Geometry: final body of the model. Coordinates: model frame, mm. A direction names the side the tool comes from. Round coordinates to 2 decimals unless told otherwise and drop trailing zeros. Loops run counter-clockwise (first coordinate to the right, second up) from the corner with the lowest first, then second, coordinate; pieces in that order, holes last. Notation, with made-up numbers: M 62.25,-9 L 120.25,-9 A19 cw 120.25,-3 Z; hole C 88.25,-6 d10. An arc over 180 degrees is marked long. Write each question's results on one line, items separated by ' | '.
```python
from build123d import *

# Parameters (mm, degrees)
SKETCH1_R           = 13
SKETCH1_R_2         = 9.5
SKETCH1_R_3         = 0.4
BOSS_EXTRUDE1_DEPTH = 1.5
BOSS_EXTRUDE2_DEPTH = 2


with BuildPart() as part:
    # Sketch1 → Boss-Extrude1 (new body)
    with BuildSketch(Plane(origin=(0, 0, 0), x_dir=(1, 0, 0), z_dir=(0, 1, 0))):
        with Locations(Location((0, 0, 0), (0, 0, 270))):
            Circle(SKETCH1_R)
        with Locations(Location((0, 0, 0), (0, 0, 270))):
            Circle(SKETCH1_R_2, mode=Mode.SUBTRACT)
        with Locations(Location((10.5, 0, 0), (0, 0, 270))):
            Circle(SKETCH1_R_3, mode=Mode.SUBTRACT)
        with Locations(Location((9.986093421, -3.244678441, 0), (0, 0, 270))):
            Circle(SKETCH1_R_3, mode=Mode.SUBTRACT)
        with Locations(Location((8.494678441, -6.171745149, 0), (0, 0, 270))):
            Circle(SKETCH1_R_3, mode=Mode.SUBTRACT)
        with Locations(Location((6.171745149, -8.494678441, 0), (0, 0, 270))):
            Circle(SKETCH1_R_3, mode=Mode.SUBTRACT)
        with Locations(Location((3.244678441, -9.986093421, 0), (0, 0, 270))):
            Circle(SKETCH1_R_3, mode=Mode.SUBTRACT)
        with Locations(Location((0, -10.5, 0), (0, 0, 270))):
            Circle(SKETCH1_R_3, mode=Mode.SUBTRACT)
        with Locations(Location((-3.244678441, -9.986093421, 0), (0, 0, 270))):
            Circle(SKETCH1_R_3, mode=Mode.SUBTRACT)
        with Locations(Location((-6.171745149, -8.494678441, 0), (0, 0, 270))):
            Circle(SKETCH1_R_3, mode=Mode.SUBTRACT)
        with Locations(Location((-8.494678441, -6.171745149, 0), (0, 0, 270))):
            Circle(SKETCH1_R_3, mode=Mode.SUBTRACT)
        with Locations(Location((-9.986093421, -3.244678441, 0), (0, 0, 270))):
            Circle(SKETCH1_R_3, mode=Mode.SUBTRACT)
        with Locations(Location((-10.5, 0, 0), (0, 0, 270))):
            Circle(SKETCH1_R_3, mode=Mode.SUBTRACT)
        with Locations(Location((-9.986093421, 3.244678441, 0), (0, 0, 270))):
            Circle(SKETCH1_R_3, mode=Mode.SUBTRACT)
        with Locations(Location((-8.494678441, 6.171745149, 0), (0, 0, 270))):
            Circle(SKETCH1_R_3, mode=Mode.SUBTRACT)
        with Locations(Location((-6.171745149, 8.494678441, 0), (0, 0, 270))):
            Circle(SKETCH1_R_3, mode=Mode.SUBTRACT)
        with Locations(Location((-3.244678441, 9.986093421, 0), (0, 0, 270))):
            Circle(SKETCH1_R_3, mode=Mode.SUBTRACT)
        with Locations(Location((0, 10.5, 0), (0, 0, 270))):
            Circle(SKETCH1_R_3, mode=Mode.SUBTRACT)
        with Locations(Location((3.244678441, 9.986093421, 0), (0, 0, 270))):
            Circle(SKETCH1_R_3, mode=Mode.SUBTRACT)
        with Locations(Location((6.171745149, 8.494678441, 0), (0, 0, 270))):
            Circle(SKETCH1_R_3, mode=Mode.SUBTRACT)
        with Locations(Location((8.494678441, 6.171745149, 0), (0, 0, 270))):
            Circle(SKETCH1_R_3, mode=Mode.SUBTRACT)
        with Locations(Location((9.986093421, 3.244678441, 0), (0, 0, 270))):
            Circle(SKETCH1_R_3, mode=Mode.SUBTRACT)
    extrude(amount=BOSS_EXTRUDE1_DEPTH)

    # Sketch2 → Boss-Extrude2 (add)
    with BuildSketch(Plane(origin=(0, 0, 0), x_dir=(1, 0, 0), z_dir=(0, 1, 0))):
        with BuildLine():
            Line((11.989578808, 0.5), (10.988630488, 0.5))
            ThreePointArc((10.988630488, 0.5), (7.778174593, 7.778174593), (0.5, 10.988630488))
            Line((0.5, 10.988630488), (0.5, 11.989578808))
            ThreePointArc((0.5, 11.989578808), (8.485281374, 8.485281374), (11.989578808, 0.5))
        make_face()
        with BuildLine():
            Line((11.989578808, -0.5), (10.988630488, -0.5))
            ThreePointArc((10.988630488, -0.5), (7.778174593, -7.778174593), (0.5, -10.988630488))
            Line((0.5, -10.988630488), (0.5, -11.989578808))
            ThreePointArc((0.5, -11.989578808), (8.485281374, -8.485281374), (11.989578808, -0.5))
        make_face()
        with BuildLine():
            Line((-0.5, -11.989578808), (-0.5, -10.988630488))
            ThreePointArc((-0.5, -10.988630488), (-7.778174593, -7.778174593), (-10.988630488, -0.5))
            Line((-10.988630488, -0.5), (-11.989578808, -0.5))
            ThreePointArc((-11.989578808, -0.5), (-8.485281374, -8.485281374), (-0.5, -11.989578808))
        make_face()
        with BuildLine():
            Line((-0.5, 10.988630488), (-0.5, 11.989578808))
            ThreePointArc((-0.5, 11.989578808), (-8.485281374, 8.485281374), (-11.989578808, 0.5))
            Line((-11.989578808, 0.5), (-10.988630488, 0.5))
            ThreePointArc((-10.988630488, 0.5), (-7.778174593, 7.778174593), (-0.5, 10.988630488))
        make_face()
    extrude(amount=-BOSS_EXTRUDE2_DEPTH)


solid = part.part
```
1. Section A-A (y = -1.2). Output: boundary loops of the cut face in (x, z), then the cut area to 3 significant figures.
Answer key:
outline: M -11.99,-0.5 A12 ccw -0.5,-11.99 L -0.5,-10.99 A11 cw -10.99,-0.5 Z; M -11.99,0.5 L -10.99,0.5 A11 cw -0.5,10.99 L -0.5,11.99 A12 ccw Z; M 0.5,-11.99 A12 ccw 11.99,-0.5 L 10.99,-0.5 A11 cw 0.5,-10.99 Z; M 0.5,10.99 A11 cw 10.99,0.5 L 11.99,0.5 A12 ccw 0.5,11.99 Z | area: 68.3 mm²
2. Section C-C (z = -7.25). Output: boundary loops of the cut face in (x, y), then the cut area to 3 significant figures.
Answer key:
outline: M -10.79,0 L -9.56,0 L -9.56,-2 L -8.27,-2 L -8.27,0 L -6.14,0 L -6.14,1.5 L -10.79,1.5 Z; M 6.14,0 L 8.27,0 L 8.27,-2 L 9.56,-2 L 9.56,0 L 10.79,0 L 10.79,1.5 L 6.14,1.5 Z | area: 19.1 mm²
3. Access query for faces 4 (the face through (-11.5, -1, 0.5)), 5 (the face through (7.858, -0.986, 7.697)), 6 (the face through (-0.5, -1, -11.5)), 7 (the face through (-7.91, 0.74, -10.316)). Directions: +Z, -Z, +X, -X, +Y, -Y. A direction counts if a zero-diameter tool reaches every point of the face in a straight line with its end or side. Return the directions, or none.
Answer key:
face 4: +X, -X, -Y | face 5: -Y | face 6: +Z, -Z, -Y | face 7: +Y, -Y
4. Section D-D (x = 7). Output: boundary loops of the cut face in (y, z), then the cut area to 3 significant figures.
Answer key:
outline: M -2,-9.75 L 0,-9.75 L 0,-10.95 L 1.5,-10.95 L 1.5,-6.42 L 0,-6.42 L 0,-8.49 L -2,-8.49 Z; M -2,8.49 L 0,8.49 L 0,6.42 L 1.5,6.42 L 1.5,10.95 L 0,10.95 L 0,9.75 L -2,9.75 Z | area: 18.6 mm²
5. Pin query (flat end, axial travel): P1, Ø0.8, axis at y = -1.5, z = -11.5, coming from the +X side; P2, Ø2, axis at y = 1, z = 3, coming from the +X side; P3, Ø1.5, axis at x = 1.5, z = 7.5, coming from the +Y side; P4, Ø0.8, axis at y = -1.5, z = 11.5, coming from the -X side. Return the tip coordinate at first contact, or that it passes through.
Answer key:
P1: stops at x = 4.56 | P2: stops at x = 12.85 | P3: passes through | P4: stops at x = -4.56
6. Draft query along Z for faces 1 (the face through (-8.57, -0.99, 8.4)), 2 (the face through (-6.052, 0.74, 8.876)), 3 (the face through (-8, -2, -8)). Return one class per face: pulls with the +Z half, pulls with the -Z half, needs draft (parallel to the pull), parting line crosses it, or undercut.
Answer key:
face 1: pulls with the +Z half | face 2: undercut | face 3: needs draft
7. Ray query, probe 1 along X at (y, z) = (-1.85, 9.25); probe 2 along Z at (x, y) = (3.75, 0.9); probe 3 along Y at (x, z) = (-8, 6.5). Return the intervals inside material, ascending.
Answer key:
probe 1: x = -7.64 to -5.95, 5.95 to 7.64 | probe 2: z = -12.45 to -8.73, 8.73 to 12.45 | probe 3: y = 0 to 1.5
8. Section B-B (x = 0). Output: boundary loops of the cut face in (y, z).
Answer key:
outline: M 0,-13 L 1.5,-13 L 1.5,-10.9 L 0,-10.9 Z; M 0,-10.1 L 1.5,-10.1 L 1.5,-9.5 L 0,-9.5 Z; M 0,9.5 L 1.5,9.5 L 1.5,10.1 L 0,10.1 Z; M 0,10.9 L 1.5,10.9 L 1.5,13 L 0,13 Z
